Build history of the part. All positions in model axes, mm. Face numbers are marked on the shaded views. A direction names the side the tool comes from. Round coordinates to 2 decimals unless told otherwise and drop trailing zeros. Loops run counter-clockwise (first coordinate to the right, second up) from the corner with the lowest first, then second, coordinate; pieces in that order, holes last. Notation, with made-up numbers: (46.5, 77.25) - (62.5, 77.25) arc R16 cw to (62.5, 102.25) - close; hole circle Ø7 at (71, 72). An arc over 180 degrees is marked (long way). Use a Markdown table: item, result.
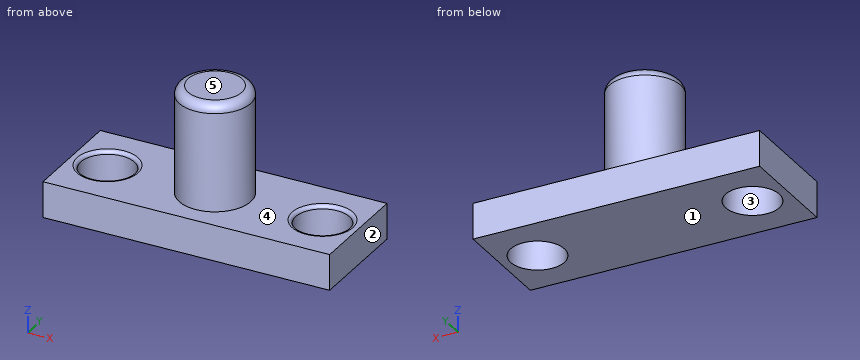
from build123d import *

# Parameters (mm, degrees)
SKETCH4_W               = 160
SKETCH4_H               = 60
BOSS_EXTRUDE1_DEPTH     = 20
SKETCH6_R               = 20
BOSS_EXTRUDE2_DEPTH     = 80
BOSS_EXTRUDE3_OUTLINE_R = 15
BOSS_EXTRUDE3_DEPTH     = 20
FILLET3_R               = 5
FILLET4_R               = 2
FILLET5_R               = 2


# Read off the part's stored shape, not the designer's step: Boss-Extrude3
with BuildPart() as part:
    # Sketch4 → Boss-Extrude1 (new body)
    with BuildSketch(Plane.XY):
        Rectangle(SKETCH4_W, SKETCH4_H)
    extrude(amount=BOSS_EXTRUDE1_DEPTH)

    # Sketch6 → Boss-Extrude2 (add)
    with BuildSketch(Plane.XY):
        with Locations(Location((0, 0, 0), (0, 0, 180))):
            Circle(SKETCH6_R)
    extrude(amount=BOSS_EXTRUDE2_DEPTH)

    # Boss-Extrude3 outline → Boss-Extrude3 (cut)
    with BuildSketch(Plane.XY):
        with Locations((60, 0)):
            Circle(BOSS_EXTRUDE3_OUTLINE_R)
        with Locations((-60, 0)):
            Circle(BOSS_EXTRUDE3_OUTLINE_R)
    extrude(amount=BOSS_EXTRUDE3_DEPTH, mode=Mode.SUBTRACT)

    # Fillet3
    fillet3_edges = [part.edges().sort_by_distance(p)[0] for p in [
        (20, 0, 80),
    ]]
    fillet(fillet3_edges, radius=FILLET3_R)

    # Fillet4
    fillet4_edges = [part.edges().sort_by_distance(p)[0] for p in [
        (-75, 0, 20),
    ]]
    fillet(fillet4_edges, radius=FILLET4_R)

    # Fillet5
    fillet5_edges = [part.edges().sort_by_distance(p)[0] for p in [
        (45, 0, 20),
    ]]
    fillet(fillet5_edges, radius=FILLET5_R)


solid = part.part
Q1. Pull direction X, two halves, no side cores. Call the marked faces 1, 2 and 3: pulls with the +X half, pulls with the -X half, needs draft (parallel to the pull), parting line crosses it, or undercut.
Results found:
| item | result |
|---|---|
| face 1 | needs draft |
| face 2 | pulls with the +X half |
| face 3 | undercut |
Q2. Cut at A-A, the plane x = -60. List the corners of the cut face in (y, z), plus the area to 3 significant figures.
Results found:
| item | result |
|---|---|
| outline | (-30, 0) - (-15, 0) - (-15, 18) arc R2 ccw to (-17, 20) - (-30, 20) - close; (15, 0) - (30, 0) - (30, 20) - (17, 20) arc R2 ccw to (15, 18) - close |
| area | 598 mm2 |
Q3. Cut at C-C, the plane z = 6. List the corners of the cut face in (x, y).
Results found:
| item | result |
|---|---|
| outline | (-80, -30) - (80, -30) - (80, 30) - (-80, 30) - close; hole circle Ø30 at (-60, 0); hole circle Ø30 at (60, 0) |
Q4. Which spindle directions (+Z, -Z, +X, -X, +Y, -Y) get a long thin tool onto all of the face, cutting with end or side? Do the marked faces 4 and 5. Say none if no direction does.
Results found:
| item | result |
|---|---|
| face 4 | +Z |
| face 5 | +Z, +X, -X, +Y, -Y |
Q5. Cut at D-D, the plane x = 0. List the corners of the cut face in (y, z).
Results found:
| item | result |
|---|---|
| outline | (-30, 0) - (30, 0) - (30, 20) - (20, 20) - (20, 75) arc R5 ccw to (15, 80) - (-15, 80) arc R5 ccw to (-20, 75) - (-20, 20) - (-30, 20) - close |
Q6. Cut at B-B, the plane y = 0. List the corners of the cut face in (x, z), plus the area to 3 significant figures.
Results found:
| item | result |
|---|---|
| outline | (-80, 0) - (-75, 0) - (-75, 18) arc R2 ccw to (-77, 20) - (-80, 20) - close; (-45, 0) - (45, 0) - (45, 18) arc R2 ccw to (43, 20) - (20, 20) - (20, 75) arc R5 ccw to (15, 80) - (-15, 80) arc R5 ccw to (-20, 75) - (-20, 20) - (-43, 20) arc R2 ccw to (-45, 18) - close; (75, 0) - (80, 0) - (80, 20) - (77, 20) arc R2 ccw to (75, 18) - close |
| area | 4,390 mm2 |
Q7. Probe line 1 (Y direction, x = -60, z = 4); line 2 (X direction, y = -3, z = 16.5); line 3 (Z direction, x = -33.5, y = -1). List the from-to ranges inside material, lowest first.
Results found:
| item | result |
|---|---|
| line 1 | y = -30 to -15, 15 to 30 |
| line 2 | x = -80 to -74.7, -45.3 to 45.3, 74.7 to 80 |
| line 3 | z = 0 to 20 |
Q8. Drop flat-ended pins along their axis: pin 1 (12 mm diameter, centred on y = 4, z = 39.5, fed in from +X); pin 2 (2 mm diameter, centred on y = 13, z = 42.5, fed in from -X); pin 3 (8 mm diameter, centred on x = 9, z = 36, fed in from -Y). Give the stop position or say it passes through.
Results found:
| item | result |
|---|---|
| pin 1 | stops at x = 20 |
| pin 2 | stops at x = -16 |
| pin 3 | stops at y = -19.36 |
